from build123d import *

# Parameters (mm, degrees)
F0_W     = 556.2346
F0_H     = 556.2346
F1_DEPTH = 12.7
F2_SIZE  = 5.08
F3_SIZE  = 5.08
F4_SIZE  = 5.08
F5_SIZE  = 5.08


with BuildPart() as f1:
    # F0 (on Front) → F1 (new body)
    with BuildSketch(Plane.XZ):
        with Locations((10.775876, 39.033592)):
            Rectangle(F0_W, F0_H)
    extrude(amount=F1_DEPTH)

    # F2
    f2_edges = [f1.edges().sort_by_distance(p)[0] for p in [
        (10.775876, 0, 317.150892),
    ]]
    chamfer(f2_edges, length=F2_SIZE)

    # F3
    f3_edges = [f1.edges().sort_by_distance(p)[0] for p in [
        (288.893176, 0, 36.493592),
    ]]
    chamfer(f3_edges, length=F3_SIZE)

    # F4
    f4_edges = [f1.edges().sort_by_distance(p)[0] for p in [
        (8.235876, 0, -239.083708),
    ]]
    chamfer(f4_edges, length=F4_SIZE)

    # F5
    f5_edges = [f1.edges().sort_by_distance(p)[0] for p in [
        (-267.341424, 0, 39.033592),
    ]]
    chamfer(f5_edges, length=F5_SIZE)


solid = f1.part
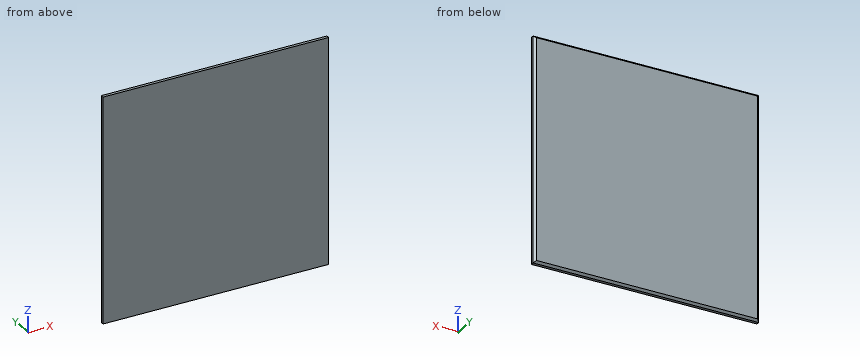
Work out the finished part from the listing and answer in its coordinate system (mm). Give positions to 0.01 mm unless a question says otherwise; leave off trailing zeros. Order: outer loops, then holes, each group sorted by start corner. A loop starts at its lowest first (then second) coordinate and runs counter-clockwise, first axis right, second up. Notation, with made-up numbers: (78.25, -24.5) - (135.25, -24.5) arc R22 cw to (135.25, -14.5) - close; hole circle Ø6 at (40.25, -12). An arc over 180 degrees is marked (long way). Answer as CSV lines item,"result". Start each with the question number.
Q1. Given pin 1 Ø2 at (y, z) = (-4, 183) entering from -X; pin 2 Ø2 at (y, z) = (-3, 236) entering from -X, each flat-ended and moving along its own axis, determine where each tip first touches the part or whether it passes through.
Q2. The part is cut by section A-A (y = -2.25). Write down the section's boundary in (x, z), then the cut area to 3 significant figures.
Q3. Find the intervals of material crossed by L1, parallel to Z at x = -166, y = -5; L2, parallel to X at y = -4.5, z = 36; L3, parallel to Z at x = 146, y = -4, in increasing order. Write a range as [from, to].
Check result:
1,pin 1,"stops at x = -267.26"
1,pin 2,"stops at x = -266.26"
2,outline,"(-264.51, -236.25) - (286.06, -236.25) - (286.06, 314.32) - (-264.51, 314.32) - close"
2,area,"303,000 mm²"
3,L1,"z = [-239, 317.07]"
3,L2,"x = [-266.76, 288.31]"
3,L3,"z = [-238, 316.07]"
